Autodesk Inventor part; units mm, degrees
ref_plane "YZ Plane" through (0, 0, 0) normal (1, 0, 0) x (0, 1, 0)
ref_plane "XZ Plane" through (0, 0, 0) normal (0, 1, 0) x (-1, 0, 0)
ref_plane "XY Plane" through (0, 0, 0) normal (0, 0, 1) x (1, 0, 0)
sketch "スケッチ1" plane through (0, 0, 0) normal (0, 0, 1) x (1, 0, 0)
  circle A0 centre (0, 0) radius 1.25
  arc A1 (0.6267, -3.189) -> (0.6267, 3.189) centre (0, 0) ccw
  line L0 (0, 0) -> (-4.5, 0)
  line L1 (-4.5, -4.1965) -> (-4.5, -4)
  line L2 (-4.5, 4) -> (-3.5, 4)
  line L3 (-3.5, 4) -> (0.6267, 3.189)
  line L4 (-4.5, -4) -> (-3.5, -4)
  line L5 (-3.5, -4) -> (0.6267, -3.189)
  line L6 (-4.5, 4) -> (-6.5, 4)
  line L7 (-4.5, -4) -> (-6.5, -4)
  line L8 (-9, 7) -> (-9, -7)
  line L9 (-9, -7) -> (-6.5, -7)
  line L10 (-9, 7) -> (-6.5, 7)
  line L11 (-6.5, 7) -> (-6.5, 4)
  line L12 (-6.5, -4) -> (-6.5, -7)
  dimension "d0" = 2.5
  dimension "d3" = 8
  dimension "d5" = 8
  dimension "d6" = 2
  dimension "d7" = 2
  dimension "d8" = 3
  dimension "d14" = 1
  dimension "d17" = 3
  dimension "d32" = 14
  dimension "d33" = 2.5
  dimension "d35" = 2
extrude "押し出し1" add sketch "スケッチ1" along normal blind 3
sketch "スケッチ2" plane through (0, 0, 3) normal (0, 0, 1) x (1, 0, 0)
  line L0 (-6.5, 7) -> (-6.5, 4)
  circle A0 centre (-6, -4.9233) radius 1.05
  circle A1 centre (-6, 4.9233) radius 1.05
  point P0 (-4.5, 4)
  point P1 (-4.5, -4)
  dimension "d13" = 2.1
  dimension "d12" = 2.1
  dimension "d15" = 0.5
extrude "押し出し2" cut sketch "スケッチ2" against normal blind 3
sketch "スケッチ4" plane through (0, 0, 3) normal (0, 0, 1) x (1, 0, 0)
  line L0 (-9, -7) -> (-9, 7)
  line L1 (-3.5, -4) -> (-5.5, -4)
  line L2 (0.6267, -3.189) -> (-3.5, -4)
  line L3 (-3.5, 4) -> (0.6267, 3.189)
  line L4 (-5.5, 4) -> (-3.5, 4)
  circle A0 centre (0, 0) radius 1.25
  line L5 (-7, 2) -> (-2.5617, 2)
  line L6 (-2.5617, -2) -> (-7, -2)
  line L7 (-7, -2) -> (-7, 2)
  arc A1 (-2.5617, 2) -> (-2.5617, -2) centre (0, 0) ccw
  arc A2 (0.6267, -3.189) -> (0.6267, 3.189) centre (0, 0) ccw
  dimension "d23" = 2
  dimension "d24" = 2
  dimension "d25" = 2
extrude "押し出し3" cut sketch "スケッチ4" against normal blind 3 contours L5 A1 L6 L7
fillet "フィレット1" radius 1 4 edges at (-2.5617, -2, 1.5) (-2.5617, 2, 1.5) (-7, -2, 1.5) (-7, 2, 1.5)
properties part number "アームユニット底板締結パーツ3t用" material "アルミニウム 2014-T4"
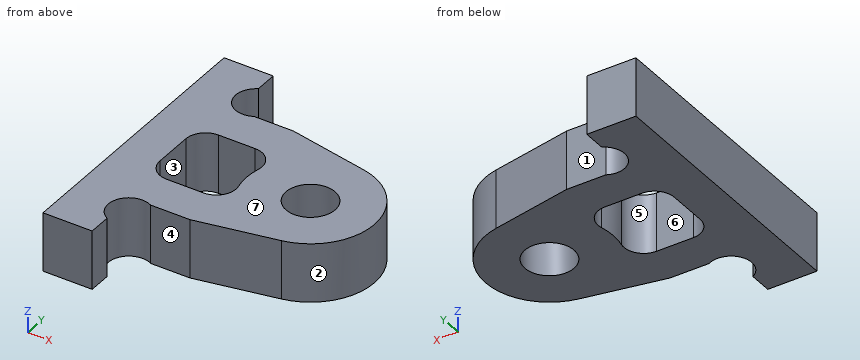
Work out the finished part from the listing and answer in its coordinate system (mm). Face numbers are marked on the shaded views. A direction names the side the tool comes from. Coordinates: 2 decimals unless noted, no trailing zeros. Write each loop counter-clockwise with the first axis right and the second up, starting at its lowest first coordinate (ties: lowest second). Pieces come first, ordered by that corner, then holes. Notation, with made-up numbers: M 33,-25.5 L 56,-25.5 A29 cw 56,6.5 Z; hole C 18.25,74 d1. An arc over 180 degrees is marked long. Use one line per item in the form item = value. Start each with the question number.
1. Straight lines are drawn through the part: probe 1 along Y at (x, z) = (-6, 2.9); probe 2 along X at (y, z) = (0.25, 1.5); probe 3 along X at (y, z) = (1, 0.6). For each, find the intervals that lie inside material, in ascending order. Write a range as from..to.
2. Each of these flat-tipped pins is pushed along its axis until it touches: P1, Ø1, axis at x = -4.5, z = 1, coming from the -Y side; P2, Ø1.5, axis at x = 0, y = 0, coming from the +Z side; P3, Ø0.6, axis at x = -4.5, z = 1, coming from the +Y side; P4, Ø0.9, axis at y = 6.5, z = 1, coming from the +X side. Where does it stop, or does it pass through?
3. The mould has two halves that part along Y. Classify the marked faces 4, 5, 6 and 7: released by +Y, released by -Y, zero draft, split by the parting line, or undercut.
4. The part is cut by section C-C (z = 2.5). Give the vertices of the cut face in (x, y).
5. The part is cut by section D-D (x = 0). Give the vertices of the cut face in (y, z).
6. The part is cut by section B-B (x = -5). Give the vertices of the cut face in (y, z).
7. The part is cut by section A-A (y = 0). Give the vertices of the cut face in (x, z).
8. A tool of negligible diameter and unlimited length cuts with its end or side. For the marked faces 1, 2 and 3, from which of +Z, -Z, +X, -X, +Y, -Y can it reach the whole face along a straight path? Write none if from no direction.
Evaluation:
q1.probe_1 = -3.87..-2, 2..3.87
q1.probe_2 = -9..-7, -3.24..-1.22, 1.22..3.24
q1.probe_3 = -9..-7, -3.13..-0.75, 0.75..3.09
q2.P1 = -4
q2.P2 = through
q2.P3 = 4
q2.P4 = -6.5
q3.face_4 = released by -Y
q3.face_5 = undercut
q3.face_6 = undercut
q3.face_7 = zero draft
q4.outline = M -9,-7 L -6.5,-7 L -6.5,-5.85 A1.05 cw -5.5,-4 L -3.5,-4 L 0.63,-3.19 A3.25 ccw 0.63,3.19 L -3.5,4 L -5.5,4 A1.05 cw -6.5,5.85 L -6.5,7 L -9,7 Z; hole M -7,-1 A1 ccw -6,-2 L -4.13,-2 A1 ccw -3.16,-0.76 A3.25 cw -3.16,0.76 A1 ccw -4.13,2 L -6,2 A1 ccw -7,1 Z; hole C 0,0 d2.5
q5.outline = M -3.31,0 L -1.25,0 L -1.25,3 L -3.31,3 Z; M 1.25,0 L 3.31,0 L 3.31,3 L 1.25,3 Z
q6.outline = M -4,0 L -2,0 L -2,3 L -4,3 Z; M 2,0 L 4,0 L 4,3 L 2,3 Z
q7.outline = M -9,0 L -7,0 L -7,3 L -9,3 Z; M -3.25,0 L -1.25,0 L -1.25,3 L -3.25,3 Z; M 1.25,0 L 3.25,0 L 3.25,3 L 1.25,3 Z
q8.face_1 = +Z, -Z, +X, +Y
q8.face_2 = +Z, -Z, +X
q8.face_3 = +Z, -Z
